Can you work these out from the model? Positions are in its coordinate system, mm. A direction names the side the tool comes from. Coordinates: 2 decimals unless noted, no trailing zeros. Loops run counter-clockwise (first coordinate to the right, second up) from the corner with the lowest first, then second, coordinate; pieces in that order, holes last.
```python
from build123d import *

# Parameters (mm, degrees)
F0_W     = 120.65
F0_H     = 50.8
F1_DEPTH = 9.525
F2_R     = 3.175
F4_D     = 5.1054
F4_DEPTH = 12.7
F4_TIP   = 1.5338169022


with BuildPart() as f1:
    # F0 (on Right) → F1 (new body, symmetric)
    with BuildSketch(Plane.YZ):
        Rectangle(F0_W, F0_H)
    extrude(amount=F1_DEPTH, both=True)

    # F2
    f2_edges = [f1.edges().sort_by_distance(p)[0] for p in [
        (0, -60.325, 25.4),
        (0, 60.325, 25.4),
    ]]
    fillet(f2_edges, radius=F2_R)

    # F4
    with Locations(Plane(origin=(0, 0, -25.4), x_dir=(1, 0, 0), z_dir=(0, 0, -1))):
        with Locations((0, 38.1), (0, 0), (0, -38.1)):
            Hole(F4_D / 2, depth=F4_DEPTH)
            with Locations((0, 0, -(F4_DEPTH + F4_TIP / 2))):  # 118° drill point
                Cone(0, F4_D / 2, F4_TIP, mode=Mode.SUBTRACT)


solid = f1.part
```
(1) I want a section at A-A on z = -17. Write out the boundary of the cut face in (x, y) (3 decimals).
Check values:
outline: (-9.525, -60.325) - (9.525, -60.325) - (9.525, 60.325) - (-9.525, 60.325) - close; hole circle Ø5.105 at (0, -38.1); hole circle Ø5.105 at (0, 0); hole circle Ø5.105 at (0, 38.1)
(2) If we mould it in two halves opening along X, with no side actions, what happens to faces 3 (the flat face through (4, -1, -25.4)), 4 (the conical face through (0.42, -0.13, -11.43)), 5 (the conical face through (-0.1, -37.67, -11.43)), 6 (the flat face through (9.525, -1, 0))? For each: released by +X, released by -X, zero draft, split by the parting line, or undercut.
Check values:
face 3: zero draft
face 4: undercut
face 5: undercut
face 6: released by +X
(3) Which directions (+Z, -Z, +X, -X, +Y, -Y) give clear straight access to the entire face, cutting with the end or side of a thin tool? Please do faces 1 (the flat face through (0, -60.325, -2)), 2 (the cylindrical face through (0.33, 35.57, -18.96)).
Check values:
face 1: +Z, -Z, +X, -X, -Y
face 2: -Z
(4) I'm going to push a flat-ended pin straight in: pin 1 (4.5 mm diameter, centred on x = 0, y = 38.1, fed in from -Z). Where does the tip first touch, or does it pass through?
Check values:
pin 1: stops at z = -12.52
(5) If I drill on probe 1 along Y at (x, z) = (0, -15.5) (3 decimals); probe 2 along X at (y, z) = (38.1, -18.75) (3 decimals); probe 3 along Y at (x, z) = (-2, -21.5) (3 decimals), over which ranges is the centre line in solid material (lowest first)?
Check values:
probe 1: y = -60.325 to -40.653, -35.547 to -2.553, 2.553 to 35.547, 40.653 to 60.325
probe 2: x = -9.525 to -2.553, 2.553 to 9.525
probe 3: y = -60.325 to -39.686, -36.514 to -1.586, 1.586 to 36.514, 39.686 to 60.325
